Here's how the part is built. I have some questions about the finished solid (model axes, mm). Face numbers are marked on the shaded views. Give positions to 0.01 mm unless a question says otherwise; leave off trailing zeros. Write each loop counter-clockwise with the first axis right and the second up, starting at its lowest first coordinate (ties: lowest second). Pieces come first, ordered by that corner, then holes. Notation, with made-up numbers: (58.5, 56.25) -> (107.5, 56.25) arc R12 cw to (107.5, 73.25) -> close; hole circle Ø10 at (77, 68.5). An arc over 180 degrees is marked (long way). Put each result on its own line as item: value. Start each with the question number.
Autodesk Inventor part; units mm, degrees
ref_plane "YZ Plane" through (0, 0, 0) normal (1, 0, 0) x (0, 1, 0)
ref_plane "XZ Plane" through (0, 0, 0) normal (0, 1, 0) x (-1, 0, 0)
ref_plane "XY Plane" through (0, 0, 0) normal (0, 0, 1) x (1, 0, 0)
sketch "Sketch1" plane through (0, 0, 0) normal (0, 1, 0) x (-1, 0, 0)
  arc A0 (6.3027, -103.9963) -> (-6.3005, -104.0126) centre (0, -103.172) ccw
  arc A1 (-4.4356, -132.0932) -> (4.4356, -132.6708) centre (0, -132.382) ccw
  line L0 (6.3563, -103.172) -> (4.4356, -132.6708)
  line L1 (-6.3563, -103.172) -> (-4.4356, -132.0932)
  point P0 (0, 0)
  dimension "d0" = 12.7127
  dimension "d1" = 8.89
  dimension "d2" = 29.21
extrude "Extrusion1" add sketch "Sketch1" along normal blind 2.794 contours L0 A1 L1 A0
sketch "Sketch2" plane through (0, 0, 0) normal (0, -1, 0) x (1, 0, 0)
  circle A0 centre (0, -103.172) radius 4.445
  arc A1 (6.3563, -103.172) -> (-6.3563, -103.172) centre (0, -103.172) ccw
  point P0 (0, 0)
  dimension "d5" = 8.89
  dimension "d6" = 0
extrude "Extrusion2" add sketch "Sketch2" along normal blind 4.064
shell "Shell1" thickness 1.27 removed faces 1 at (-0.8417, -4.064, -105.7685)
sketch "Sketch3" plane through (0, 2.794, 0) normal (0, 1, 0) x (1, 0, 0)
  circle A0 centre (0, 132.636) radius 0.635
  circle A1 centre (0, 129.842) radius 0.635
  circle A2 centre (0, 127.048) radius 0.635
  circle A3 centre (0, 124.254) radius 0.635
  circle A4 centre (0, 121.46) radius 0.635
  circle A5 centre (0, 118.666) radius 0.635
  arc A6 (4.4356, 132.0932) -> (-4.4356, 132.6708) centre (0, 132.382) ccw
  arc A7 (-6.3563, 103.172) -> (6.3563, 103.172) centre (0, 103.172) ccw
  point P0 (0, 0)
  dimension "d10" = 1.27
  dimension "d11" = 1.27
  dimension "d12" = 1.27
  dimension "d13" = 1.27
  dimension "d14" = 1.27
  dimension "d15" = 1.27
  dimension "d16" = 2.794
  dimension "d17" = 2.794
  dimension "d18" = 2.794
  dimension "d19" = 2.794
  dimension "d20" = 2.794
  dimension "d22" = 15.494
extrude "Extrusion3" cut sketch "Sketch3" against normal blind 4.064
sketch "Sketch4" plane through (0, 2.794, 0) normal (0, 1, 0) x (1, 0, 0)
  circle A0 centre (0, 103.172) radius 3.175
  circle A1 centre (0, 103.172) radius 3.175
  point P0 (0, 0)
extrude "Extrusion4" cut sketch "Sketch4" against normal blind 0.508
equation "\"d11\" = d10"
equation "\"d12\" = d11"
equation "\"d13\" = d12"
equation "\"d14\" = d10"
equation "\"d15\" = d10"
equation "\"d17\" = d16"
equation "\"d18\" = d17"
equation "\"d19\" = d18"
equation "\"d20\" = d19"
properties part number "Servo Horn"
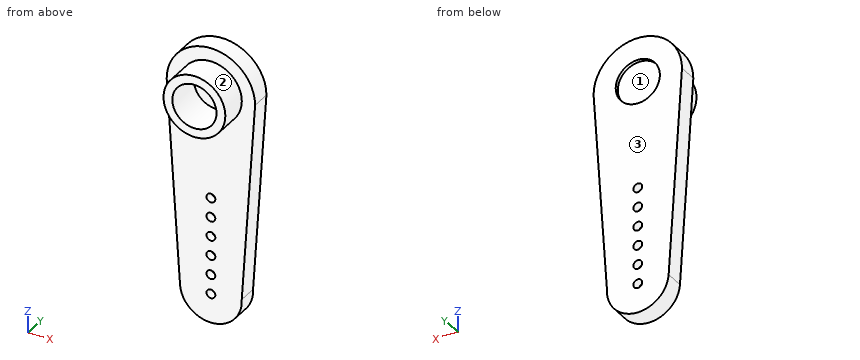
1) Thinking about a two-plate mould opening in Z: for the marked faces 1, 2 and 3, which applies, released by +Z, released by -Z, zero draft, split by the parting line, or undercut?
2) I want a section at D-D, the plane y = -3.5. Write out the boundary of the cut face in (x, z) (3 decimals), and give its area (3 significant figures).
3) I need wall thicknesses on probe 1 along Y at (x, z) = (3, -132); probe 2 along Y at (x, z) = (2.5, -106); probe 3 along Y at (x, z) = (-5.5, -106). Which ranges of each line are inside material? Lowest first, please.
4) I want a section at C-C, the plane x = -3.75. Write out the boundary of the cut face in (y, z), and give its area (3 significant figures).
5) I want a section at A-A, the plane z = -121.46. Write out the boundary of the cut face in (x, y) (3 decimals), and give its area (3 significant figures).
6) I want a section at B-B, the plane x = 0. State how many separate pieces and enclosed holes the cut face has, and give its area (3 significant figures).
7) I'm going to push flat-ended pins straight in: pin 1 Ø1.5 at (y, z) = (-1, -103.5) entering from +X (3 decimals); pin 2 Ø3 at (x, y) = (2, -2) entering from -Z; pin 3 Ø1.7 at (x, z) = (0, -129.842) entering from -Y; pin 4 Ø0.8 at (x, z) = (0, -132.636) entering from -Y. Where does each tip first touch, or does it pass through?
Established:
1. face 1: undercut
1. face 2: split by the parting line
1. face 3: zero draft
2. outline: circle Ø8.89 at (0, -103.172); hole circle Ø6.35 at (0, -103.172)
2. area: 30.4 mm2
3. probe 1: y = 0 to 1.27, 1.52 to 2.79
3. probe 2: y = -4.06 to 1.27, 1.52 to 2.79
3. probe 3: y = 0 to 2.79
4. outline: (-4.06, -105.56) -> (0, -105.56) -> (0, -134.77) -> (2.79, -134.77) -> (2.79, -98.04) -> (0, -98.04) -> (0, -100.79) -> (-4.06, -100.79) -> close; hole (1.27, -123.65) -> (1.52, -123.65) -> (1.52, -99.74) -> (1.27, -99.74) -> close
4. area: 116 mm2
5. outline: (-5.166, 0) -> (-0.635, 0) -> (-0.635, 1.27) -> (-3.893, 1.27) -> (-3.893, 1.524) -> (-0.635, 1.524) -> (-0.635, 2.794) -> (-5.166, 2.794) -> close; (0.635, 0) -> (5.142, 0) -> (5.142, 2.794) -> (0.635, 2.794) -> (0.635, 1.524) -> (3.869, 1.524) -> (3.869, 1.27) -> (0.635, 1.27) -> close
5. area: 23.6 mm2
6. separate pieces: 13
6. enclosed holes: 0
6. area: 82.0 mm2
7. pin 1: stops at x = 4.445
7. pin 2: stops at z = -107.59
7. pin 3: stops at y = 0
7. pin 4: passes through
